Read the model definition and answer for the solid it produces. Units are mm, in the model's axes. A direction names the side the tool comes from. Coordinates: 2 decimals unless noted, no trailing zeros. Loops run counter-clockwise (first coordinate to the right, second up) from the corner with the lowest first, then second, coordinate; pieces in that order, holes last. Notation, with made-up numbers: (53, 13) -> (107, 13) arc R18 cw to (107, 33) -> close; hole circle Ø11 at (18, 16.5). An arc over 180 degrees is marked (long way). Answer as a JSON object with one key per item and string values. Group by question number.
Q1. Each of these flat-tipped pins is pushed along its axis until it touches: P1, Ø3, axis at x = -12, z = -165, coming from the +Y side; P2, Ø6, axis at x = -8.5, z = -149, coming from the -Y side; P3, Ø12, axis at y = -90, z = -221.5, coming from the -X side. Where does it stop, or does it pass through?
Q2. Determine the mould class of faces 4 (the flat face through (3.62, -69, -179)), 5 (the flat face through (-13, 2.032, -148)), 6 (the flat face through (2.318, -56.329, -200.444)), 7 (the cylindrical face through (2.815, -85.344, -187.748)) for opening direction Y: released by +Y, released by -Y, zero draft, split by the parting line, or undercut.
Q3. The part is cut by section C-C on z = -190.5. Write down the section's boundary in (x, y).
Q4. The part is cut by section D-D on z = -159.5. Write down the section's boundary in (x, y).
Q5. The part is cut by section B-B on x = -10.5. Write down the section's boundary in (y, z).
Q6. For faces 1 (the flat face through (2.032, -67, -196)), 2 (the flat face through (2.837, -124.286, -224.18)), 3 (the cylindrical face through (-9.87, 2.84, -133.67)), determine the directions among +Z, -Z, +X, -X, +Y, -Y from which every point of the face is accessible in a straight line to the end or side of a thin tool.
Q7. Straight lines are drawn through the part: line 1 along Y through (x, z) = (2.5, -192); line 2 along X through (y, z) = (-125.5, -215.5). For each, find the intervals that lie inside material, in ascending order. Write a range as [from, to].
Q8. The part is cut by section A-A on y = -41. Write down the section's boundary in (x, z), and give its area (3 significant figures).
from build123d import *

# Parameters (mm, degrees)
SKETCH1_R                = 4.064
BOSS_EXTRUDE1_DEPTH      = 2.032
SKETCH2_R                = 4.064
BOSS_EXTRUDE2_DEPTH      = 2.032
FILLET1_R                = 2.032
BOSS_EXTRUDE3_DEPTH      = 58.42
BOSS_EXTRUDE3_DEPTH_BACK = 239.395
CUT_EXTRUDE1_DEPTH       = 1
CUT_EXTRUDE1_DEPTH_BACK  = 483.6
CUT_EXTRUDE2_DEPTH       = 25.4475
SKETCH7_R                = 4.064
CUT_EXTRUDE3_DEPTH       = 25.4475
SKETCH8_R                = 4.064
CUT_EXTRUDE4_DEPTH       = 136.562269206
SKETCH10_R               = 10.67677981
SKETCH10_R_2             = 9.251177106
SKETCH10_R_3             = 9.294395921
SKETCH10_R_4             = 10.207707861
SKETCH10_R_5             = 7.460626698
SKETCH10_R_6             = 11.174016497
CUT_EXTRUDE5_DEPTH       = 2.5875


with BuildPart() as part:
    # Sketch1 → Boss-Extrude1 (new body)
    with BuildSketch(Plane(origin=(0, 0, 0), x_dir=(0, 0, -1), z_dir=(1, 0, 0))):
        Polygon((-193.675, 0), (193.675, 0), (239.395, -132.715), (239.395, -161.29), (-243.205, -161.29), (-243.205, -132.715), align=None)
        with Locations((219.075, -116.84)):
            Circle(SKETCH1_R, mode=Mode.SUBTRACT)
    extrude(amount=BOSS_EXTRUDE1_DEPTH)

    # Sketch2 → Boss-Extrude2 (add)
    with BuildSketch(Plane(origin=(0, 0, 0), x_dir=(1, 0, 0), z_dir=(0, 1, 0))):
        Polygon((2.032, -193.675), (2.032, 193.675), (0, 193.675), (-20.828, 165.1), (-20.828, -165.1), (0, -193.675), align=None)
        with Locations((-9.779, -32.7025)):
            Circle(SKETCH2_R, mode=Mode.SUBTRACT)
        with BuildLine():
            Line((-13.843, 144.8435), (-13.843, 137.7315))
            ThreePointArc((-13.843, 137.7315), (-9.779, 133.6675), (-5.715, 137.7315))
            Line((-5.715, 137.7315), (-5.715, 144.8435))
            ThreePointArc((-5.715, 144.8435), (-9.779, 148.9075), (-13.843, 144.8435))
        make_face(mode=Mode.SUBTRACT)
    extrude(amount=BOSS_EXTRUDE2_DEPTH)

    # Fillet1
    fillet1_edges = [part.edges().sort_by_distance(p)[0] for p in [
        (2.032, 2.032, 0),
    ]]
    fillet(fillet1_edges, radius=FILLET1_R)

    # Sketch3 → Boss-Extrude3 (add, two sides)
    with BuildSketch(Plane.XY) as boss_extrude3_sk:
        with BuildLine():
            Line((-1.376033354, 2.032), (-20.828, 2.032))
            Line((-20.828, 2.032), (-20.828, 3.6195))
            Line((-20.828, 3.6195), (3.6195, 3.6195))
            Line((3.6195, 3.6195), (3.6195, -161.29))
            Line((3.6195, -161.29), (2.032, -161.29))
            Line((2.032, -161.29), (2.032, -132.715))
            Line((2.032, -132.715), (2.032, -1.376033354))
            ThreePointArc((2.032, -1.376033354), (1.735294181, 1.735294181), (-1.376033354, 2.032))
        make_face()
    extrude(amount=BOSS_EXTRUDE3_DEPTH)
    extrude(boss_extrude3_sk.sketch, amount=-BOSS_EXTRUDE3_DEPTH_BACK)

    # Sketch4 → Cut-Extrude1 (cut, two sides)
    with BuildSketch(Plane(origin=(0, 0, -239.395), x_dir=(-1, 0, 0), z_dir=(0, 0, -1))) as cut_extrude1_sk:
        with BuildLine():
            Line((0, -161.29), (44.263147165, -161.29))
            Line((44.263147165, -161.29), (44.263147165, 7.390927462))
            Line((44.263147165, 7.390927462), (27.636319643, 7.390927462))
            Line((27.636319643, 7.390927462), (27.636319643, 2.032))
            Line((27.636319643, 2.032), (1.376033354, 2.032))
            ThreePointArc((1.376033354, 2.032), (-1.735294181, 1.735294181), (-2.032, -1.376033354))
            Line((-2.032, -1.376033354), (-2.032, -132.715))
            Line((-2.032, -132.715), (-2.032, -161.29))
            Line((-2.032, -161.29), (0, -161.29))
        make_face()
    extrude(amount=CUT_EXTRUDE1_DEPTH, mode=Mode.SUBTRACT)
    extrude(cut_extrude1_sk.sketch, amount=-CUT_EXTRUDE1_DEPTH_BACK, mode=Mode.SUBTRACT)

    # Sketch6 → Cut-Extrude2 (cut, through all)
    with BuildSketch(Plane(origin=(3.6195, 0, 0), x_dir=(0, 0, -1), z_dir=(1, 0, 0))):
        Polygon((164.593410128, 3.6195), (236.630427362, -116.84), (211.375744463, -131.942769206), (130.306990873, 3.6195), (-58.42, 3.6195), (-58.42, -161.29), (239.395, -161.29), (239.395, 3.6195), align=None)
    extrude(amount=-CUT_EXTRUDE2_DEPTH, mode=Mode.SUBTRACT)

    # Sketch7 → Cut-Extrude3 (cut, through all)
    with BuildSketch(Plane(origin=(3.6195, 0, 0), x_dir=(0, 0, -1), z_dir=(1, 0, 0))):
        with Locations((219.075, -116.84)):
            Circle(SKETCH7_R)
    extrude(amount=-CUT_EXTRUDE3_DEPTH, mode=Mode.SUBTRACT)

    # Sketch8 → Cut-Extrude4 (cut, through all)
    with BuildSketch(Plane(origin=(0, 3.6195, 0), x_dir=(1, 0, 0), z_dir=(0, 1, 0))):
        with Locations((-9.779, -32.7025)):
            Circle(SKETCH8_R)
        with BuildLine():
            Line((-13.843, 144.8435), (-13.843, 137.7315))
            ThreePointArc((-13.843, 137.7315), (-9.779, 133.6675), (-5.715, 137.7315))
            Line((-5.715, 137.7315), (-5.715, 144.8435))
            ThreePointArc((-5.715, 144.8435), (-9.779, 148.9075), (-13.843, 144.8435))
        make_face()
    extrude(amount=-CUT_EXTRUDE4_DEPTH, mode=Mode.SUBTRACT)

    # Sketch10 → Cut-Extrude5 (cut, through all)
    with BuildSketch(Plane.ZY.offset(-2.032)):
        with Locations((-210.642167036, -101.738031393)):
            Circle(SKETCH10_R)
        with Locations((-186.895001779, -60.948782833)):
            Circle(SKETCH10_R_2)
        with Locations((-175.719865187, -42.509807457)):
            Circle(SKETCH10_R_3)
        with Locations((-163.706593351, -23.512075251)):
            Circle(SKETCH10_R_4)
        with Locations((-149.737672611, -10.381289755)):
            Circle(SKETCH10_R_5)
        with Locations((-198.07013837, -81.064028698)):
            Circle(SKETCH10_R_6)
    extrude(amount=-CUT_EXTRUDE5_DEPTH, mode=Mode.SUBTRACT)


solid = part.part
Final values:
{
 "1": {"P1": "stops at y = 3.62", "P2": "stops at y = 2.03", "P3": "stops at x = 2.03"},
 "2": {"face 4": "zero draft", "face 5": "released by -Y", "face 6": "released by +Y", "face 7": "undercut"},
 "3": {"outline": "(2.03, -97.03) -> (3.62, -97.03) -> (3.62, -89.28) -> (2.03, -89.28) -> close; (2.03, -72.85) -> (3.62, -72.85) -> (3.62, -69.47) -> (2.03, -69.47) -> close; (2.03, -52.43) -> (3.62, -52.43) -> (3.62, -39.7) -> (2.03, -39.7) -> close"},
 "4": {"outline": "(-20.83, 2.03) -> (-1.38, 2.03) arc R2.45 cw to (2.03, -1.38) -> (2.03, -14.21) -> (3.62, -14.21) -> (3.62, 3.62) -> (-20.83, 3.62) -> close; (2.03, -45.2) -> (3.62, -45.2) -> (3.62, -32.81) -> (2.03, -32.81) -> close"},
 "5": {"outline": "(2.03, -165.54) -> (3.62, -164.59) -> (3.62, -148.84) -> (2.03, -148.84) -> close; (2.03, -133.73) -> (3.62, -133.73) -> (3.62, -130.31) -> (2.03, -131.26) -> close"},
 "6": {"face 1": "+Z, -Z, -X, -Y", "face 2": "-Z, +X, -X, -Y", "face 3": "+Y, -Y"},
 "7": {"line 1": "y = [-99.54, -90.45], [-71.68, -68.66], [-53.23, -42.21]", "line 2": "x = [2.03, 3.62]"},
 "8": {"outline": "(2.03, -191.28) -> (3.62, -191.28) -> (3.62, -184.89) -> (2.03, -184.89) -> close; (2.03, -166.55) -> (3.62, -166.55) -> (3.62, -156.99) -> (2.03, -156.99) -> close", "area": "25.3 mm2"}
}
